from build123d import *

# Parameters (mm, degrees)
SKETCH1_W           = 48.35
SKETCH1_H           = 24.35
BOSS_EXTRUDE1_DEPTH = 13.7
SKETCH2_R           = 0.5
SKETCH2_W           = 22
SKETCH2_H           = 11.5
CUT_EXTRUDE1_DEPTH  = 1
SKETCH3_W           = 5
SKETCH3_H           = 6.5
CUT_EXTRUDE2_DEPTH  = 1
SKETCH4_R           = 0.75
SKETCH4_W           = 1.5
SKETCH4_H           = 1.5
CUT_EXTRUDE3_DEPTH  = 1
SKETCH5_W           = 5
SKETCH5_H           = 6.5
CUT_EXTRUDE4_DEPTH  = 1
SKETCH6_R           = 1
SKETCH6_W           = 7
SKETCH6_H           = 24.35
CUT_EXTRUDE5_DEPTH  = 2.5
SKETCH7_W           = 10
SKETCH7_H           = 5.15
CUT_EXTRUDE6_DEPTH  = 1
FILLET1_R           = 3


with BuildPart() as part:
    # Sketch1 → Boss-Extrude1 (new body)
    with BuildSketch(Plane(origin=(0, 0, 0), x_dir=(1, 0, 0), z_dir=(0, 1, 0))):
        with Locations((24.175, 12.175)):
            Rectangle(SKETCH1_W, SKETCH1_H)
    extrude(amount=BOSS_EXTRUDE1_DEPTH)

    # Sketch2 → Cut-Extrude1 (cut)
    with BuildSketch(Plane(origin=(0, 13.7, 0), x_dir=(1, 0, 0), z_dir=(0, 1, 0))):
        with Locations(Location((46.35, 19.35, 0), (0, 0, 270))):
            Circle(SKETCH2_R)
        with BuildLine():
            Line((6.5, 19.85), (6.5, 4.5))
            Line((6.5, 4.5), (13.5, 4.5))
            ThreePointArc((13.5, 4.5), (14.914213562, 5.085786438), (15.5, 6.5))
            Line((15.5, 6.5), (15.5, 17.85))
            ThreePointArc((15.5, 17.85), (14.914213562, 19.264213562), (13.5, 19.85))
            Line((13.5, 19.85), (6.5, 19.85))
        make_face()
        with Locations((32.65, 12.2)):
            Rectangle(SKETCH2_W, SKETCH2_H)
    extrude(amount=-CUT_EXTRUDE1_DEPTH, mode=Mode.SUBTRACT)

    # Sketch3 → Cut-Extrude2 (cut)
    with BuildSketch(Plane(origin=(0, 0, -24.35), x_dir=(-1, 0, 0), z_dir=(0, 0, -1))):
        with Locations((-9.5, 7.95)):
            Rectangle(SKETCH3_W, SKETCH3_H)
    extrude(amount=-CUT_EXTRUDE2_DEPTH, mode=Mode.SUBTRACT)

    # Sketch4 → Cut-Extrude3 (cut)
    with BuildSketch(Plane(origin=(48.35, 0, 0), x_dir=(0, 0, -1), z_dir=(1, 0, 0))):
        with Locations((19.35, 8.7)):
            Circle(SKETCH4_R)
        with Locations((5.828571429, 1.27)):
            Rectangle(SKETCH4_W, SKETCH4_H)
        with Locations((3.29, 1.27)):
            Rectangle(SKETCH4_W, SKETCH4_H)
        with Locations((8.367142857, 1.27)):
            Rectangle(SKETCH4_W, SKETCH4_H)
        with Locations((10.905714286, 1.27)):
            Rectangle(SKETCH4_W, SKETCH4_H)
        with Locations((13.444285714, 1.27)):
            Rectangle(SKETCH4_W, SKETCH4_H)
        with Locations((15.982857143, 1.27)):
            Rectangle(SKETCH4_W, SKETCH4_H)
        with Locations((18.521428571, 1.27)):
            Rectangle(SKETCH4_W, SKETCH4_H)
        with Locations((21.06, 1.27)):
            Rectangle(SKETCH4_W, SKETCH4_H)
    extrude(amount=-CUT_EXTRUDE3_DEPTH, mode=Mode.SUBTRACT)

    # Sketch5 → Cut-Extrude4 (cut)
    with BuildSketch(Plane.XY):
        with Locations((31.35, 7.45)):
            Rectangle(SKETCH5_W, SKETCH5_H)
    extrude(amount=-CUT_EXTRUDE4_DEPTH, mode=Mode.SUBTRACT)

    # Sketch6 → Cut-Extrude5 (cut)
    with BuildSketch(Plane.XZ):
        with Locations(Location((9, -4, 0), (0, 0, 270))):
            Circle(SKETCH6_R)
        with Locations(Location((9, -20.35, 0), (0, 0, 270))):
            Circle(SKETCH6_R)
        with Locations((3.5, -12.175)):
            Rectangle(SKETCH6_W, SKETCH6_H)
    extrude(amount=-CUT_EXTRUDE5_DEPTH, mode=Mode.SUBTRACT)

    # Sketch7 → Cut-Extrude6 (cut)
    with BuildSketch(Plane.ZY):
        with BuildLine():
            Line((-15.175, 11.7), (-9.175, 11.7))
            ThreePointArc((-9.175, 11.7), (-7.675, 10.2), (-9.175, 8.7))
            Line((-9.175, 8.7), (-15.175, 8.7))
            ThreePointArc((-15.175, 8.7), (-16.675, 10.2), (-15.175, 11.7))
        make_face()
        with Locations((-12.175, 5.075)):
            Rectangle(SKETCH7_W, SKETCH7_H)
    extrude(amount=-CUT_EXTRUDE6_DEPTH, mode=Mode.SUBTRACT)

    # Fillet1
    # the kernel refuses this fillet: 3 mm, written as the material it takes off along each edge
    with BuildSketch(Plane(origin=(0, -5, -24.35), x_dir=(0, 0, 1), z_dir=(0, 1, 0)), Plane(origin=(0, -5, 0), x_dir=(1, 0, 0), z_dir=(0, 1, 0))) as fillet1_piece_1:
        with BuildLine():
            CenterArc((FILLET1_R, FILLET1_R), FILLET1_R, 180, 90)
            Line((0, FILLET1_R), (0, 0))
            Line((0, 0), (FILLET1_R, 0))
        make_face()
    extrude(amount=26.2, mode=Mode.SUBTRACT)
    with BuildSketch(Plane(origin=(48.35, -7.5, -24.35), x_dir=(0, 0, 1), z_dir=(0, 1, 0)), Plane(origin=(48.35, -7.5, 0), x_dir=(-1, 0, 0), z_dir=(0, 1, 0))) as fillet1_piece_2:
        with BuildLine():
            CenterArc((FILLET1_R, -FILLET1_R), FILLET1_R, 90, 90)
            Line((0, -FILLET1_R), (0, 0))
            Line((0, 0), (FILLET1_R, 0))
        make_face()
    extrude(amount=28.7, mode=Mode.SUBTRACT)


solid = part.part
Here's how the part is built. I have some questions about the finished solid (model axes, mm). A direction names the side the tool comes from. Round coordinates to 2 decimals unless told otherwise and drop trailing zeros. Loops run counter-clockwise (first coordinate to the right, second up) from the corner with the lowest first, then second, coordinate; pieces in that order, holes last. Notation, with made-up numbers: M 82.5,-25 L 113.5,-25 A17 cw 113.5,3 Z; hole C -7,81 d3. An arc over 180 degrees is marked long. Write each question's results on one line, items separated by ' | '. Start each with the question number.
(1) I want a section at A-A (x = 33). Please give me the cut outline in (y, z).
(2) I want a section at C-C (x = 38). Please give me the cut outline in (y, z).
(3) If I drill on probe 1 along X at (y, z) = (1.2, -4); probe 2 along Y at (x, z) = (48.05, -19.35); probe 3 along Y at (x, z) = (22, -10.25), over which ranges is the centre line in solid material (lowest first)? Write a range as from..to.
(4) Thinking about a two-plate mould opening in Z: for faces 6 (the flat face through (48.35, 7, -12)), 7 (the flat face through (48, 1, -7.617)), 8 (the flat face through (48, 0.52, -6)), which applies, pulls with the +Z half, pulls with the -Z half, needs draft (parallel to the pull), parting line crosses it, or undercut?
(5) On a 3-axis mill with a long thin cutter (end or side, diameter ignored), from which of +Z, -Z, +X, -X, +Y, -Y can I reach the whole of each face in a straight line? I mean faces 1 (the flat face through (46.4, 12.7, -19.4)), 2 (the flat face through (12, 8, -24)), 3 (the flat face through (0.5, 5, -17.175)), 4 (the cylindrical face through (10, 1, -4)), 5 (the flat face through (48, 1, -2.54)). Say none if no direction works.
(6) I want a section at B-B (y = 10.2). Please give me the cut outline in (x, z) (3 decimals).
(7) Will these pins go through, and if not, where does the flat tip stop? P1, Ø0.5, axis at x = 46.5, z = -19.5, coming from the +Y side; P2, Ø1.1, axis at x = 48, y = 1.5, coming from the -Z side; P3, Ø1.5, axis at x = 10.5, y = 7, coming from the -Z side.
(8) I want a section at D-D (x = 4). Please give me the cut outline in (y, z), then the cut area to 3 significant figures.
Solved:
1) outline: M 0,-24.35 L 13.7,-24.35 L 13.7,-17.95 L 12.7,-17.95 L 12.7,-6.45 L 13.7,-6.45 L 13.7,0 L 10.7,0 L 10.7,-1 L 4.2,-1 L 4.2,0 L 0,0 Z
2) outline: M 0,-24.35 L 13.7,-24.35 L 13.7,-17.95 L 12.7,-17.95 L 12.7,-6.45 L 13.7,-6.45 L 13.7,0 L 0,0 Z
3) probe 1: x = 7..8, 10..47.35 | probe 2: y = 0..7.95, 9.45..13.7 | probe 3: y = 0..12.7
4) face 6: needs draft | face 7: undercut | face 8: undercut
5) face 1: +Y | face 2: -Z | face 3: -X, -Y | face 4: -Y | face 5: +X
6) outline: M 0,-21.35 A3 ccw 3,-24.35 L 7,-24.35 L 7,-23.35 L 12,-23.35 L 12,-24.35 L 45.35,-24.35 A3 ccw 48.35,-21.35 L 48.35,-3 A3 ccw 45.35,0 L 33.85,0 L 33.85,-1 L 28.85,-1 L 28.85,0 L 3,0 A3 ccw 0,-3 L 0,-7.675 L 1,-7.675 L 1,-16.675 L 0,-16.675 Z
7) P1: stops at y = 12.7 | P2: stops at z = -23.49 | P3: stops at z = -23.35
8) outline: M 2.5,-24.35 L 13.7,-24.35 L 13.7,0 L 2.5,0 Z | area: 273 mm²
